Read the model definition and answer for the solid it produces. Units are mm, in the model's axes. Face numbers are marked on the shaded views. A direction names the side the tool comes from. Round coordinates to 2 decimals unless told otherwise and drop trailing zeros. Loops run counter-clockwise (first coordinate to the right, second up) from the corner with the lowest first, then second, coordinate; pieces in that order, holes last. Notation, with made-up numbers: M -12.5,22 L 1.5,22 A21 ccw 1.5,39 Z; hole C -19.75,53 d6. An arc over 180 degrees is marked long. Write each question's results on one line, items separated by ' | '.
from build123d import *

# Parameters (mm, degrees)
SKETCH1_W           = 200
SKETCH1_H           = 200
BOSS_EXTRUDE1_DEPTH = 250
SKETCH2_W           = 210
SKETCH2_H           = 210
BOSS_EXTRUDE2_DEPTH = 5
SKETCH3_W           = 210
SKETCH3_H           = 210
BOSS_EXTRUDE3_DEPTH = 5
SKETCH4_W           = 190
SKETCH4_H           = 190
CUT_EXTRUDE1_DEPTH  = 300.416098432


with BuildPart() as part:
    # Sketch1 → Boss-Extrude1 (new body)
    with BuildSketch(Plane.XY):
        Rectangle(SKETCH1_W, SKETCH1_H)
    extrude(amount=BOSS_EXTRUDE1_DEPTH)

    # Sketch2 → Boss-Extrude2 (add)
    with BuildSketch(Plane.XY.offset(250)):
        Rectangle(SKETCH2_W, SKETCH2_H)
    extrude(amount=BOSS_EXTRUDE2_DEPTH)

    # Sketch3 → Boss-Extrude3 (add)
    with BuildSketch(Plane(origin=(0, 0, 0), x_dir=(-1, 0, 0), z_dir=(0, 0, -1))):
        Rectangle(SKETCH3_W, SKETCH3_H)
    extrude(amount=BOSS_EXTRUDE3_DEPTH)

    # Sketch4 → Cut-Extrude1 (cut, through all)
    with BuildSketch(Plane.XY.offset(255)):
        Rectangle(SKETCH4_W, SKETCH4_H)
    extrude(amount=-CUT_EXTRUDE1_DEPTH, mode=Mode.SUBTRACT)


solid = part.part
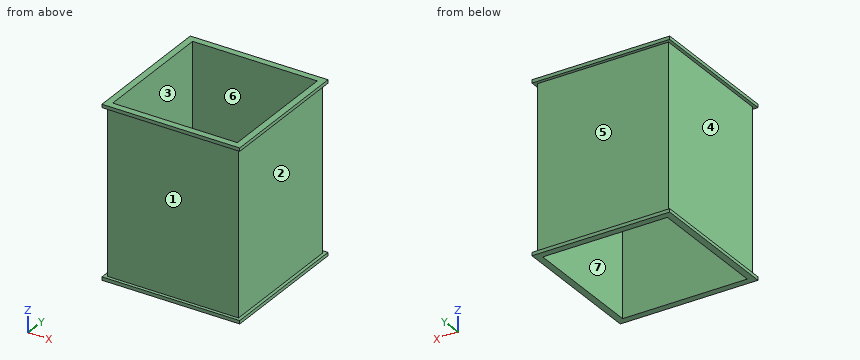
Item 1: The part is cut by section C-C (z = 124.5). Determine the outline of the cut face in (x, y).
Outcome:
outline: M -100,-100 L 100,-100 L 100,100 L -100,100 Z; hole M -95,-95 L 95,-95 L 95,95 L -95,95 Z
Item 2: The part is cut by section A-A (x = 0). Determine the outline of the cut face in (y, z), plus the area to 3 significant figures.
Outcome:
outline: M -105,-5 L -95,-5 L -95,255 L -105,255 L -105,250 L -100,250 L -100,0 L -105,0 Z; M 95,-5 L 105,-5 L 105,0 L 100,0 L 100,250 L 105,250 L 105,255 L 95,255 Z | area: 2,700 mm2
Item 3: A straight line is drawn through the part: line 1 (X direction, y = -54.5, z = 244.5). Find the intervals that lie inside material, in ascending order.
Outcome:
line 1: x = -100 to -95, 95 to 100
Item 4: The mould has two halves that part along X. Classify the marked faces 4, 5, 6 and 7: pulls with the +X half, pulls with the -X half, needs draft (parallel to the pull), parting line crosses it, or undercut.
Outcome:
face 4: pulls with the -X half | face 5: needs draft | face 6: undercut | face 7: undercut
Item 5: Flat-ended cylindrical pins translate along their axes: pin 1 (3 mm diameter, centred on y = -1, z = 140, fed in from -X); pin 2 (1 mm diameter, centred on x = 69.5, z = 207.5, fed in from +Y); pin 3 (3 mm diameter, centred on x = -78, z = 148, fed in from -Y). Find the tip coordinate at first contact, or state that the pin passes through.
Outcome:
pin 1: stops at x = -100 | pin 2: stops at y = 100 | pin 3: stops at y = -100
Item 6: For the marked faces 1, 2 and 3, determine the directions among +Z, -Z, +X, -X, +Y, -Y from which every point of the face is accessible in a straight line to the end or side of a thin tool.
Outcome:
face 1: +X, -X, -Y | face 2: +X, +Y, -Y | face 3: +Z, -Z
